Input: dimensioned drawing with shaded views. Units: mm. Origin: part minimum x, y, z. Coordinates: 2 decimals unless noted, no trailing zeros. Loops run counter-clockwise (first coordinate to the right, second up) from the corner with the lowest first, then second, coordinate; pieces in that order, holes last. Notation, with made-up numbers: M -4,13.25 L 8,13.25 A22 ccw 8,36.25 Z; hole C -20.75,-4 d7. An arc over 180 degrees is marked long. Write item = value, one per line. Start each with the question number.
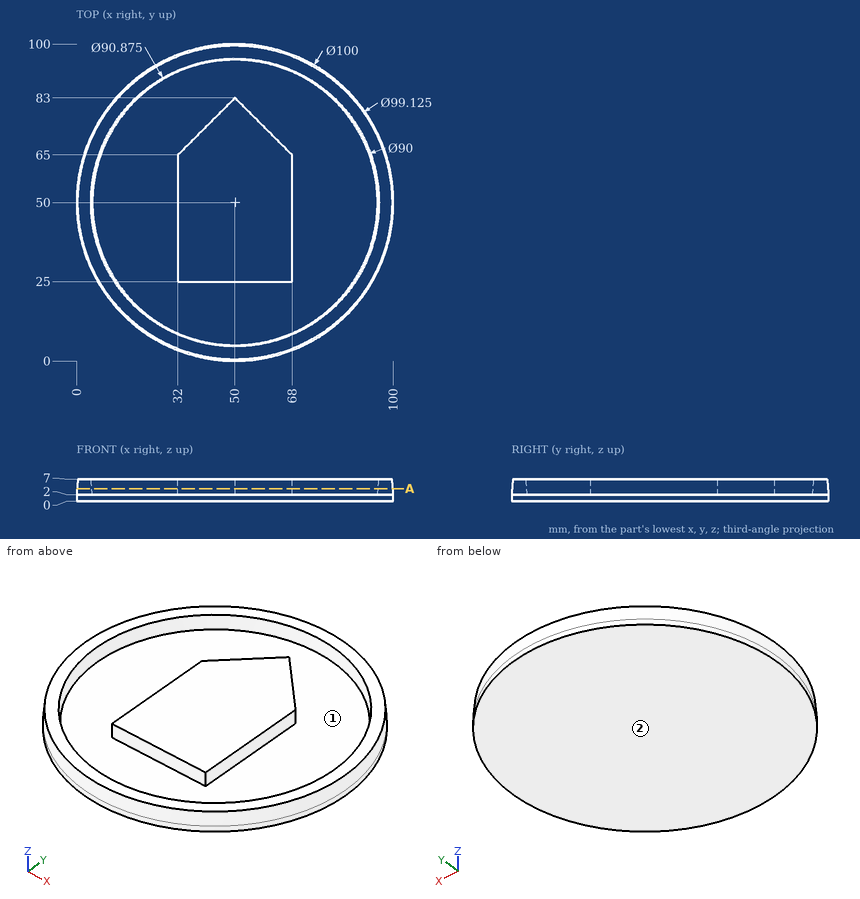
Item 1: Section query A-A (z = 4). Return the cut outline in (x, y) (3 decimals).
Item 2: First-contact query: pin 1 (1 mm diameter, centred on y = 44.5, z = 2, fed in from -X); pin 2 (3 mm diameter, centred on y = 71, z = 1.5, fed in from -X); pin 3 (1.5 mm diameter, centred on x = 75.5, z = 4.5, fed in from -Y). Flat tips, straight axial feed; report the tip coordinate or a pass-through.
Item 3: Line query: line 1 (X direction, y = 40, z = 2.25); line 2 (X direction, y = 73.5, z = 2.25); line 3 (Y direction, x = 55, z = 5.25). Output: solid intervals per line, ascending. Write a range as from..to.
Item 4: Pull-direction query (Y, two-part tool) for the marked faces 1 and 2; classes: released by +Y, released by -Y, zero draft, split by the parting line, or undercut.
Verdict:
q1.outline = C 50,50 d99.65; M 32,25 L 68,25 L 68,65 L 50,83 L 32,65 Z; hole C 50,50 d90.35
q2.pin_1 = 0.25
q2.pin_2 = 3.96
q2.pin_3 = 6.8
q3.line_1 = 1.03..6.1, 32..68, 93.9..98.97
q3.line_2 = 5.89..11.6, 40.5..59.5, 88.4..94.11
q3.line_3 = 0.54..4.99, 25..78, 95.01..99.46
q4.face_1 = undercut
q4.face_2 = zero draft
